Source: CAD feature listing. Evaluate the final solid. Frame: model axes, mm. Face numbers are marked on the shaded views. A direction names the side the tool comes from. Coordinates: 2 decimals unless noted, no trailing zeros. Order: outer loops, then holes, each group sorted by start corner. A loop starts at its lowest first (then second) coordinate and runs counter-clockwise, first axis right, second up. Notation, with made-up numbers: (-8.75, 81) -> (18.25, 81) arc R11 cw to (18.25, 92) -> close; hole circle Ø3 at (-14, 0). An arc over 180 degrees is marked (long way). Write each question's results on one line, items separated by ' | '. Start each with the question number.
from build123d import *

# Parameters (mm, degrees)
F0_R     = 6.95
F1_DEPTH = 6.6
F2_R     = 7.5
F3_DEPTH = 5
F4_R     = 6.95
F5_DEPTH = 3
F6_R     = 3
F7_DEPTH = 13


with BuildPart() as f1:
    # F0 (on Top) → F1 (new body)
    with BuildSketch(Plane.XY):
        Circle(F0_R)
    extrude(amount=F1_DEPTH)

    # F2 (on face) → F3 (join)
    with BuildSketch(Plane.XY.offset(6.6)):
        Circle(F2_R)
    extrude(amount=F3_DEPTH)

    # F4 (on face) → F5 (join)
    with BuildSketch(Plane.XY.offset(11.6)):
        Circle(F4_R)
    extrude(amount=F5_DEPTH)

    # F6 (on face) → F7 (cut)
    with BuildSketch(Plane(origin=(0, 0, 0), x_dir=(1, 0, 0), z_dir=(0, 0, -1))):
        Circle(F6_R)
    extrude(amount=-F7_DEPTH, mode=Mode.SUBTRACT)


solid = f1.part
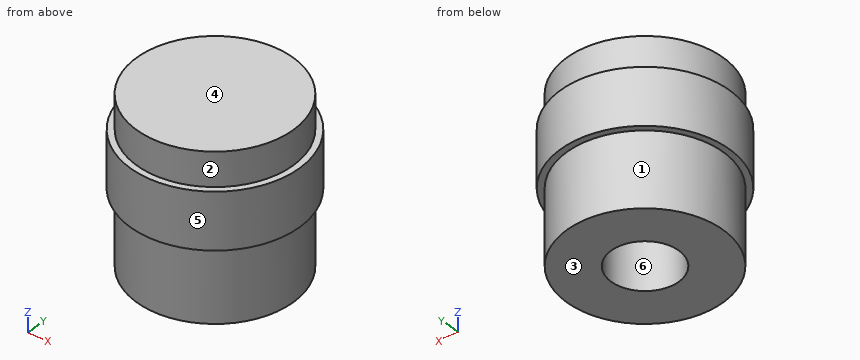
(1) Section A-A on y = 0. Return the cut outline in (x, z).
(2) First-contact query: P1, Ø1.5, axis at x = 6, z = 12.5, coming from the -Y side; P2, Ø1.8, axis at x = -1.5, y = 1, coming from the -Z side; P3, Ø5, axis at x = 1.5, z = 3, coming from the -Y side. Flat tips, straight axial feed; report the tip coordinate or a pass-through.
(3) Reachability of the marked faces 1, 2 and 3 from +Z, -Z, +X, -X, +Y, -Y: full face, straight path, thin tool, end or side. Return the list, or none.
(4) Section C-C on z = 2.75. Return the cut outline in (x, y).
(5) Draft query along Y for the marked faces 4, 5 and 6. Return one class per face: released by +Y, released by -Y, zero draft, split by the parting line, or undercut.
(6) Section D-D on x = -6. Return the cut outline in (y, z), then the cut area to 3 significant figures.
(7) Line query: L1, parallel to Y at x = 0, z = 10.25; L2, parallel to Z at x = -1, y = 2; L3, parallel to Y at x = 0, z = 4.5. Output: solid intervals per line, ascending.
Results list:
1) outline: (-7.5, 6.6) -> (-6.95, 6.6) -> (-6.95, 0) -> (-3, 0) -> (-3, 13) -> (3, 13) -> (3, 0) -> (6.95, 0) -> (6.95, 6.6) -> (7.5, 6.6) -> (7.5, 11.6) -> (6.95, 11.6) -> (6.95, 14.6) -> (-6.95, 14.6) -> (-6.95, 11.6) -> (-7.5, 11.6) -> close
2) P1: stops at y = -4.55 | P2: stops at z = 13 | P3: stops at y = -6.95
3) face 1: -Z | face 2: +Z | face 3: -Z, +X, -X, +Y, -Y
4) outline: circle Ø13.9 at (0, 0); hole circle Ø6 at (0, 0)
5) face 4: zero draft | face 5: split by the parting line | face 6: undercut
6) outline: (-4.5, 6.6) -> (-3.51, 6.6) -> (-3.51, 0) -> (3.51, 0) -> (3.51, 6.6) -> (4.5, 6.6) -> (4.5, 11.6) -> (3.51, 11.6) -> (3.51, 14.6) -> (-3.51, 14.6) -> (-3.51, 11.6) -> (-4.5, 11.6) -> close | area: 112 mm²
7) L1: y = -7.5 to -3, 3 to 7.5 | L2: z = 13 to 14.6 | L3: y = -6.95 to -3, 3 to 6.95
